Geometry: see drawing. Coordinates: mm, zero at the bounding-box minimum. Round coordinates to 2 decimals unless told otherwise and drop trailing zeros. Loops run counter-clockwise (first coordinate to the right, second up) from the corner with the lowest first, then second, coordinate; pieces in that order, holes last.
(1) Section B-B, the plane y = 10.5. Return the cut outline in (x, z), plus the area to 3 significant figures.
(2) Section A-A, the plane x = 127. Count the separate pieces of the cut face and the enclosed holes in it, plus the area to 3 significant figures.
(3) First-contact query: pin 1 Ø5.5 at (x, y) = (127, 66.675) entering from +Z; pin 2 Ø10 at (x, z) = (66.5, 15.5) entering from -Y (1 decimal). Flat tips, straight axial feed; report the tip coordinate or a pass-through.
(4) Material intervals for probe 1 along Y at (x, z) = (129, 23) (1 decimal); probe 2 along X at (y, z) = (66.5, 9); probe 3 along Y at (x, z) = (129.5, 13.5) (1 decimal), sorted ascending.
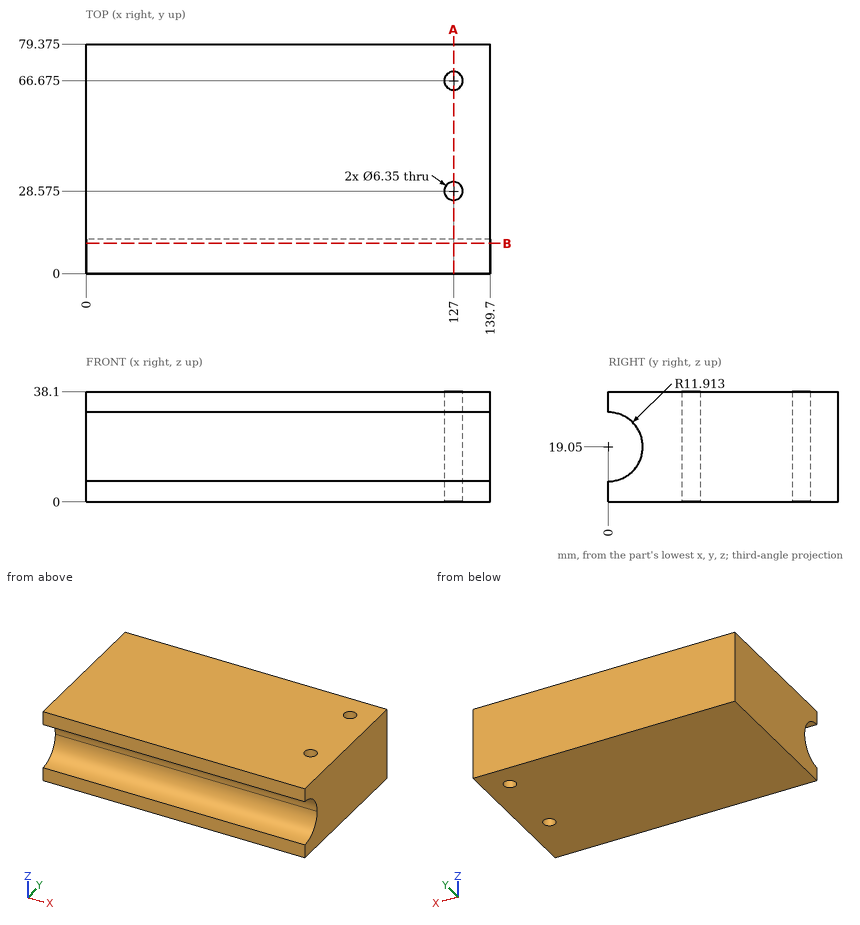
Output values:
1. outline: (0, 0) - (139.7, 0) - (139.7, 13.42) - (0, 13.42) - close; (0, 24.68) - (139.7, 24.68) - (139.7, 38.1) - (0, 38.1) - close
1. area: 3,750 mm2
2. separate pieces: 3
2. enclosed holes: 0
2. area: 2,320 mm2
3. pin 1: passes through
3. pin 2: stops at y = 8.3
4. probe 1: y = 11.2 to 26.1, 31 to 64.2, 69.1 to 79.4
4. probe 2: x = 0 to 123.83, 130.17 to 139.7
4. probe 3: y = 10.5 to 26.6, 30.5 to 64.7, 68.6 to 79.4
